```python
from build123d import *

# Parameters (mm, degrees)
SKETCH2_W                = 914.4
SKETCH2_H                = 1143
BOSS_EXTRUDE1_DEPTH      = 508
CUT_EXTRUDE1_DEPTH       = 1550.4
BOSS_EXTRUDE2_DEPTH      = 25.4
BOSS_EXTRUDE2_DEPTH_BACK = 939.8
SKETCH4_R                = 101.6
CUT_EXTRUDE2_REACH       = 1566.525
SKETCH5_W                = 736.6
SKETCH5_H                = 736.6


with BuildPart() as part:
    # Sketch2 → Boss-Extrude1 (new body)
    with BuildSketch(Plane.XY):
        with Locations((457.2, 571.5)):
            Rectangle(SKETCH2_W, SKETCH2_H)
    extrude(amount=BOSS_EXTRUDE1_DEPTH)

    # Sketch3 → Cut-Extrude1 (cut, through all)
    with BuildSketch(Plane(origin=(914.4, 0, 0), x_dir=(0, 0, -1), z_dir=(1, 0, 0))):
        Polygon((-508, 241.3), (-254, 0), (-508, 0), align=None)
    extrude(amount=-CUT_EXTRUDE1_DEPTH, mode=Mode.SUBTRACT)

    # Sketch4 → Boss-Extrude2 (add, two sides: drawn at the far end of the back side and taken through both)
    with BuildSketch(Plane(origin=(914.4, 0, 0), x_dir=(0, 0, -1), z_dir=(1, 0, 0)).offset(-BOSS_EXTRUDE2_DEPTH_BACK)):
        with Locations((-254, 910.669925226)):
            Circle(SKETCH4_R)
        with Locations((-254, 446.916916509)):
            Circle(SKETCH4_R)
    extrude(amount=BOSS_EXTRUDE2_DEPTH + BOSS_EXTRUDE2_DEPTH_BACK)

    # Sketch5 → Cut-Extrude2 (cut, up to next)
    with BuildSketch(Plane.XY.offset(508), mode=Mode.PRIVATE) as cut_extrude2_sk1:
        with Locations((457.2, 698.5)):
            Rectangle(SKETCH5_W, SKETCH5_H)
    cut_extrude2_tool1 = extrude(cut_extrude2_sk1.sketch, amount=-CUT_EXTRUDE2_REACH, mode=Mode.PRIVATE) & part.part
    add(cut_extrude2_tool1.solids().sort_by_distance((457.2, 698.5, 508))[0], mode=Mode.SUBTRACT)


solid = part.part
```
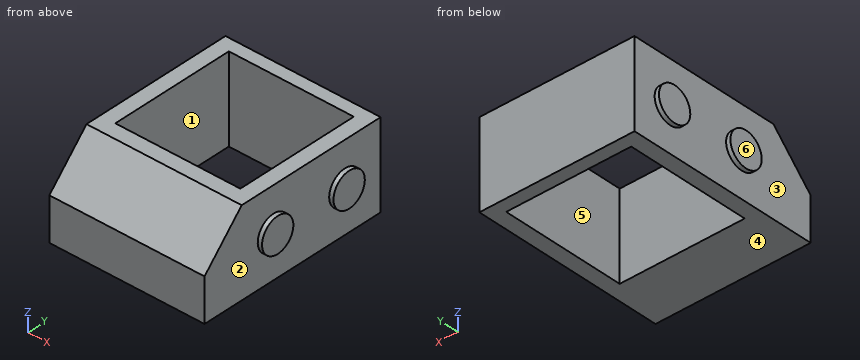
Can you work these out from the model? Positions are in its coordinate system, mm. Face numbers are marked on the shaded views. A direction names the side the tool comes from. Coordinates: 2 decimals unless noted, no trailing zeros. Order: outer loops, then holes, each group sorted by start corner. A loop starts at its lowest first (then second) coordinate and runs counter-clockwise, first axis right, second up.
1. Thinking about a two-plate mould opening in X: for the marked faces 4, 5 and 6, which applies, +X half, -X half, draft (parallel to the pull), parting line (faces both ways), or undercut?
2. If we section it at D-D (x = 52): Please give me the cut outline in (y, z).
3. If we section it at B-B (y = 359): Please give me the cut outline in (x, z), then the cut area to 3 significant figures.
4. I'm going to push flat-ended pins straight in: pin 1 (3 mm diameter, centred on y = 533, z = 340.5, fed in from -X); pin 2 (1.5 mm diameter, centred on y = 666, z = 75.5, fed in from +X). Where does each tip first touch, or does it pass through?
5. If we section it at C-C (z = 306.5): Please give me the cut outline in (x, y) (3 decimals), then the cut area to 3 significant figures.
6. For the marked faces 1, 2 and 3, which set-ups out of +Z, -Z, +X, -X, +Y, -Y let a thin tool reach every point of the face, with its end or its side?
7. I need wall thicknesses on line 1 (Y direction, x = 389, z = 187); line 2 (X direction, y = 570, z = 454); line 3 (X direction, y = 863, z = 278). Which ranges of each line are inside material? Lowest first, please.
8. If we section it at A-A (x = 634): Please give me the cut outline in (y, z), then the cut area to 3 significant figures.
Entries:
1. face 4: draft
1. face 5: undercut
1. face 6: -X half
2. outline: (0, 0) - (1143, 0) - (1143, 508) - (241.3, 508) - (0, 254) - close
3. outline: (-25.4, 203.08) - (0, 203.08) - (0, 0) - (88.9, 0) - (88.9, 508) - (0, 508) - (0, 304.92) - (-25.4, 304.92) - close; (825.5, 0) - (914.4, 0) - (914.4, 203.08) - (939.8, 203.08) - (939.8, 304.92) - (914.4, 304.92) - (914.4, 508) - (825.5, 508) - close
3. area: 95,500 mm2
4. pin 1: stops at x = 0
4. pin 2: stops at x = 914.4
5. outline: (-25.4, 359.932) - (0, 359.932) - (0, 49.875) - (914.4, 49.875) - (914.4, 359.932) - (939.8, 359.932) - (939.8, 533.901) - (914.4, 533.901) - (914.4, 823.685) - (939.8, 823.685) - (939.8, 997.654) - (914.4, 997.654) - (914.4, 1143) - (0, 1143) - (0, 997.654) - (-25.4, 997.654) - (-25.4, 823.685) - (0, 823.685) - (0, 533.901) - (-25.4, 533.901) - close; hole (88.9, 330.2) - (825.5, 330.2) - (825.5, 1066.8) - (88.9, 1066.8) - close
5. area: 475,000 mm2
6. face 1: +Z, -Z
6. face 2: +X
6. face 3: -X
7. line 1: y = 0 to 330.2, 1066.8 to 1143
7. line 2: x = 0 to 88.9, 825.5 to 914.4
7. line 3: x = -25.4 to 88.9, 825.5 to 939.8
8. outline: (0, 0) - (330.2, 0) - (330.2, 508) - (241.3, 508) - (0, 254) - close; (1066.8, 0) - (1143, 0) - (1143, 508) - (1066.8, 508) - close
8. area: 176,000 mm2
